Input: part model. Units: mm. Frame: model coordinates. A direction names the side the tool comes from. Coordinates: 2 decimals unless noted, no trailing zeros. Loops run counter-clockwise (first coordinate to the right, second up) from the corner with the lowest first, then second, coordinate; pieces in that order, holes last. Notation, with made-up numbers: (67.5, 86.5) -> (99.5, 86.5) arc R18 cw to (99.5, 108.5) -> close; hole circle Ø4 at (34, 14.25). An arc over 180 degrees is marked (long way). Put each result on its own line as item: value. Start each with the question number.
1) Pull-direction query (Y, two-part tool) for faces 6 (the cylindrical face through (597.462, -8.537, 13.325)), 7 (the conical face through (74.844, 14.667, 0.84)), 8 (the conical face through (-34.14, 1.17, 0.16)); classes: pulls with the +Y half, pulls with the -Y half, needs draft (parallel to the pull), parting line crosses it, or undercut.
2) Cut plane A-A (x = 440.5). Return the cut outline in (y, z).
3) Contact query for flat-ended pins moving along their axis: P1, Ø1, axis at x = 325.5, z = 23.5, coming from the -Y side; P2, Ø3.5, axis at x = 28.5, z = 13, coming from the +Y side; P3, Ø12, axis at y = 19.5, z = 5, coming from the -X side. Output: stop coordinate, or through.
4) Material intervals for L1, parallel to Y at x = 506, z = 3.5; L2, parallel to Y at x = 0, z = 14.5; L3, parallel to X at y = 12, z = 2.5, sorted ascending.
5) Set-up query: faces 1 (the flat face through (333, -4, 0)), 2 (the flat face through (55.985, -15.046, 13.675)), 3 (the cylindrical face through (39.629, 23.537, 13.325)), 4 (the flat face through (339, 15, 18.5)), 5 (the cylindrical face through (75, 15, 3)). Return all of +Z, -Z, +X, -X, +Y, -Y with unobstructed straight access to the full face (end or side cutting, diameter ignored); none if empty.
from build123d import *

# Parameters (mm, degrees)
EXTRUDE_1_DEPTH      = 27
SKETCH_2_R           = 20.5
CUT_EXTRUDE_1_DEPTH  = 45
CUT_EXTRUDE_2_DEPTH  = 50
EXTRUDE_2_DEPTH      = 27
CUT_EXTRUDE_3_DEPTH  = 8.5
CUT_EXTRUDE_START    = -8.5
CUT_EXTRUDE_4_DEPTH  = 8.5
CHAMFER_2_SIZE       = 1
FILLET_1_R           = 4
FILLET_2_R           = 45
EXTRUDE_START        = -27
EXTRUDE_3_DEPTH      = 27
SKETCH_13_R          = 23.5
CUT_EXTRUDE_8_DEPTH  = 24
SKETCH_14_R          = 2.5
CUT_EXTRUDE_9_DEPTH  = 20
CHAMFER_3_SIZE       = 0.5
CHAMFER_4_SIZE       = 1
SKETCH_15_R          = 4
CUT_EXTRUDE_10_DEPTH = 20
SKETCH_16_R          = 4
CUT_EXTRUDE_11_DEPTH = 20


with BuildPart() as part:
    # 草图1 → 拉伸1 (new body)
    with BuildSketch(Plane.XY):
        with BuildLine():
            Line((0, 22.5), (670, 22.5))
            ThreePointArc((670, 22.5), (692.5, 0), (670, -22.5))
            Line((670, -22.5), (0, -22.5))
            ThreePointArc((0, -22.5), (-22.5, 0), (0, 22.5))
        make_face()
    extrude(amount=EXTRUDE_1_DEPTH)

    # 草图2 → 切除-拉伸1 (cut)
    with BuildSketch(Plane.XY.offset(27)):
        Circle(SKETCH_2_R)
        with Locations((670, 0)):
            Circle(SKETCH_2_R)
    extrude(amount=-CUT_EXTRUDE_1_DEPTH, mode=Mode.SUBTRACT)

    # 草图3 → 切除-拉伸2 (cut)
    with BuildSketch(Plane.XY.offset(27)):
        Polygon((40, -22.5), (72.167603808, -7.5), (597.832396192, -7.5), (630, -22.5), align=None)
    extrude(amount=-CUT_EXTRUDE_2_DEPTH, mode=Mode.SUBTRACT)

    # 草图4 → 拉伸2 (add)
    with BuildSketch(Plane.XY.offset(27)):
        Polygon((630, 22.5), (40, 22.5), (72.167603808, 37.5), (597.832396192, 37.5), align=None)
    extrude(amount=-EXTRUDE_2_DEPTH)

    # 草图5 → 切除-拉伸3 (cut)
    with BuildSketch(Plane.XY.offset(27)):
        with BuildLine():
            Line((90, 30), (580, 30))
            ThreePointArc((580, 30), (595, 15), (580, 0))
            Line((580, 0), (90, 0))
            ThreePointArc((90, 0), (75, 15), (90, 30))
        make_face()
    extrude(amount=-CUT_EXTRUDE_3_DEPTH, mode=Mode.SUBTRACT)

    # 草图7 → 切除-拉伸4 (cut)
    with BuildSketch(Plane(origin=(0, 0, 0), x_dir=(-1, 0, 0), z_dir=(0, 0, -1)).offset(CUT_EXTRUDE_START)):
        with BuildLine():
            Line((-90, 30), (-580, 30))
            ThreePointArc((-580, 30), (-595, 15), (-580, 0))
            Line((-580, 0), (-90, 0))
            ThreePointArc((-90, 0), (-75, 15), (-90, 30))
        make_face()
    extrude(amount=CUT_EXTRUDE_4_DEPTH, mode=Mode.SUBTRACT)

    # 倒角2
    chamfer_2_edges = [part.edges().sort_by_distance(p)[0] for p in [
        (75, 15, 27),
        (335, 0, 27),
        (595, 15, 27),
        (335, 30, 27),
        (75, 15, 0),
        (335, 30, 0),
        (595, 15, 0),
        (335, 0, 0),
    ]]
    chamfer(chamfer_2_edges, length=CHAMFER_2_SIZE)

    # 圆角1
    fillet_1_edges = [part.edges().sort_by_distance(p)[0] for p in [
        (75, 15, 18.5),
        (335, 30, 18.5),
        (595, 15, 18.5),
        (335, 0, 18.5),
        (75, 15, 8.5),
        (335, 0, 8.5),
        (595, 15, 8.5),
        (335, 30, 8.5),
    ]]
    fillet(fillet_1_edges, radius=FILLET_1_R)

    # 圆角2
    fillet_2_edges = [part.edges().sort_by_distance(p)[0] for p in [
        (630, -22.5, 13.5),
        (40, -22.5, 13.5),
        (72.167603808, -7.5, 13.5),
        (597.832396192, -7.5, 13.5),
        (597.832396192, 37.5, 13.5),
        (630, 22.5, 13.5),
        (40, 22.5, 13.5),
        (72.167603808, 37.5, 13.5),
    ]]
    fillet(fillet_2_edges, radius=FILLET_2_R)

    # 草图8 → 拉伸3 (add)
    with BuildSketch(Plane.XY.offset(27).offset(EXTRUDE_START)):
        with BuildLine():
            Line((0, 22.5), (26.809513237, 22.5))
            ThreePointArc((26.809513237, 22.5), (-35, 0), (26.809513237, -22.5))
            Line((26.809513237, -22.5), (0, -22.5))
            ThreePointArc((0, -22.5), (-22.5, 0), (0, 22.5))
        make_face()
        with BuildLine():
            Line((670, 22.5), (643.190486763, 22.5))
            ThreePointArc((643.190486763, 22.5), (705, 0), (643.190486763, -22.5))
            Line((643.190486763, -22.5), (670, -22.5))
            ThreePointArc((670, -22.5), (692.5, 0), (670, 22.5))
        make_face()
    extrude(amount=EXTRUDE_3_DEPTH)

    # 草图13 → 切除-拉伸8 (cut)
    with BuildSketch(Plane.XY.offset(27)):
        Circle(SKETCH_13_R)
        with Locations((670, 0)):
            Circle(SKETCH_13_R)
    extrude(amount=-CUT_EXTRUDE_8_DEPTH, mode=Mode.SUBTRACT)

    # 草图14 → 切除-拉伸9 (cut)
    with BuildSketch(Plane.XY.offset(27)):
        with Locations((-25.980762114, -15)):
            Circle(SKETCH_14_R)
        with Locations((644.019237886, -15)):
            Circle(SKETCH_14_R)
        with Locations((670, -30)):
            Circle(SKETCH_14_R)
        with Locations((644.019237886, 15)):
            Circle(SKETCH_14_R)
        with Locations((670, 30)):
            Circle(SKETCH_14_R)
        with Locations((-25.980762114, 15)):
            Circle(SKETCH_14_R)
        with Locations((0, 30)):
            Circle(SKETCH_14_R)
        with Locations((0, -30)):
            Circle(SKETCH_14_R)
        with Locations((25.980762114, 15)):
            Circle(SKETCH_14_R)
        with Locations((25.980762114, -15)):
            Circle(SKETCH_14_R)
        with Locations((695.980762114, 15)):
            Circle(SKETCH_14_R)
        with Locations((695.980762114, -15)):
            Circle(SKETCH_14_R)
    extrude(amount=-CUT_EXTRUDE_9_DEPTH, mode=Mode.SUBTRACT)

    # 倒角3
    chamfer_3_edges = [part.edges().sort_by_distance(p)[0] for p in [
        (646.5, 0, 27),
    ]]
    chamfer(chamfer_3_edges, length=CHAMFER_3_SIZE)

    # 倒角4
    chamfer_4_edges = [part.edges().sort_by_distance(p)[0] for p in [
        (335, -7.5, 27),
        (335, -7.5, 0),
        (613.916198096, -15, 27),
        (613.916198096, -15, 0),
        (56.083801904, -15, 27),
        (641.583373291, -22.5, 27),
        (613.916198096, 30, 27),
        (335, 37.5, 27),
        (56.083801904, 30, 27),
        (28.416626709, 22.5, 27),
        (72.404080999, 36.43332032, 27),
        (39.763522808, -21.43332032, 27),
        (597.595919001, 36.43332032, 27),
        (630.236477192, -21.43332032, 27),
        (641.583373291, -22.5, 0),
        (56.083801904, -15, 0),
        (28.416626709, 22.5, 0),
        (56.083801904, 30, 0),
        (335, 37.5, 0),
        (613.916198096, 30, 0),
        (72.404080999, 36.43332032, 0),
        (39.763522808, -21.43332032, 0),
        (597.595919001, 36.43332032, 0),
        (630.236477192, -21.43332032, 0),
        (597.595919001, -8.56667968, 27),
        (597.595919001, -8.56667968, 0),
        (630.236477192, 23.56667968, 27),
        (630.236477192, 23.56667968, 0),
        (39.763522808, 23.56667968, 27),
        (39.763522808, 23.56667968, 0),
        (72.404080999, -8.56667968, 27),
        (72.404080999, -8.56667968, 0),
        (28.416626709, -22.5, 0),
        (28.416626709, -22.5, 27),
        (-35, 0, 0),
        (-35, 0, 27),
        (641.583373291, 22.5, 0),
        (641.583373291, 22.5, 27),
        (705, 0, 0),
        (705, 0, 27),
    ]]
    chamfer(chamfer_4_edges, length=CHAMFER_4_SIZE)

    # 草图15 → 切除-拉伸10 (cut)
    with BuildSketch(Plane.XZ.offset(7.5)):
        with Locations((320, 13.5)):
            Circle(SKETCH_15_R)
        with Locations((360, 13.5)):
            Circle(SKETCH_15_R)
    extrude(amount=-CUT_EXTRUDE_10_DEPTH, mode=Mode.SUBTRACT)

    # 草图16 → 切除-拉伸11 (cut)
    with BuildSketch(Plane(origin=(0, 0, 0), x_dir=(-1, 0, 0), z_dir=(0, 0, -1))):
        with Locations((-54.94315244, -2.5)):
            Circle(SKETCH_16_R)
        with Locations((-55, 17.499919209)):
            Circle(SKETCH_16_R)
    extrude(amount=-CUT_EXTRUDE_11_DEPTH, mode=Mode.SUBTRACT)


solid = part.part
Results found:
1. face 6: pulls with the -Y half
1. face 7: undercut
1. face 8: parting line crosses it
2. outline: (-7.5, 1) -> (-6.5, 0) -> (-1, 0) -> (0, 1) -> (0, 4.5) arc R4 cw to (4, 8.5) -> (26, 8.5) arc R4 cw to (30, 4.5) -> (30, 1) -> (31, 0) -> (36.5, 0) -> (37.5, 1) -> (37.5, 26) -> (36.5, 27) -> (31, 27) -> (30, 26) -> (30, 22.5) arc R4 cw to (26, 18.5) -> (4, 18.5) arc R4 cw to (0, 22.5) -> (0, 26) -> (-1, 27) -> (-6.5, 27) -> (-7.5, 26) -> close
3. P1: stops at y = -7.5
3. P2: stops at y = 22.57
3. P3: stops at x = -32.29
4. L1: y = -7.5 to 0, 30 to 37.5
4. L2: y = -35 to -32.5, -27.5 to -23.5, 23.5 to 27.5, 32.5 to 35
4. L3: x = -32.88 to -16.62, 16.62 to 75.3, 594.7 to 653.38, 686.62 to 702.88
5. face 1: -Z, +X, -X, +Y, -Y
5. face 2: +Z, -Z, -Y
5. face 3: +Z, -Z, +Y
5. face 4: +Z
5. face 5: -Z
